Model file for the job. Use its own axes, mm. A direction names the side the tool comes from. Give positions to 0.01 mm unless a question says otherwise; leave off trailing zeros. Loops run counter-clockwise (first coordinate to the right, second up) from the corner with the lowest first, then second, coordinate; pieces in that order, holes last. Notation, with made-up numbers: M -14.5,-37 L 39.5,-37 A23 cw 39.5,-3 Z; hole C 27.25,58.5 d4. An arc over 180 degrees is marked long. Answer in a Markdown table with one row per item.
```python
from build123d import *

# Parameters (mm, degrees)
REVOLUTION001_ANGLE = 16
FILLET_R            = 6


with BuildPart() as part:
    # Sketch → Revolution (revolve)
    with BuildSketch(Plane.XZ):
        with BuildLine():
            ThreePointArc((42.295694, 49.859657), (40.314757, 47.066424), (39.35, 43.780773))
            Line((44.35, 43.780773), (39.35, 43.780773))
            Line((47.827156, 53.147992), (44.35, 43.780773))
            Line((42.827156, 53.147992), (47.827156, 53.147992))
            Line((42.827156, 51.147992), (42.827156, 53.147992))
            ThreePointArc((42.295694, 49.859657), (42.689073, 50.451167), (42.827156, 51.147992))
        make_face()
    revolve(axis=Axis((0, 0, 0), (0, 0, 1)))

    # Sketch004 → Revolution001 (revolve, symmetric)
    with BuildSketch(Plane.XZ) as revolution001_sk:
        with BuildLine():
            Line((44.35, 43.780773), (44.072018, 50.32))
            Line((44.072018, 50.32), (47.83229, 53.160461))
            Line((47.83229, 53.160461), (50.83229, 53.160461))
            Line((50.83229, 53.160461), (50.83229, 65.160461))
            Line((50.83229, 65.160461), (60.83229, 65.160461))
            Line((60.83229, 65.160461), (60.83229, 53.160461))
            add(Edge.make_bspline(
                [(50.83229, 43.780773), (60.83229, 43.780773), (60.83229, 53.160461)],
                knots=[4.712389, 4.712389, 4.712389, 6.283185, 6.283185, 6.283185], degree=2, weights=[1, 0.707107, 1]))
            Line((50.83229, 43.780773), (44.35, 43.780773))
        make_face()
    revolve(axis=Axis((0, 0, 0), (0, 0, 1)), revolution_arc=REVOLUTION001_ANGLE / 2)
    revolve(revolution001_sk.sketch, axis=Axis((0, 0, 0), (0, 0, -1)), revolution_arc=REVOLUTION001_ANGLE / 2)

    # Sketch003 → Groove (revolve, cut)
    with BuildSketch(Plane(origin=(51, 0, 59), x_dir=(-1, 0, 0), z_dir=(0, -1, 0))):
        Polygon((0, 5), (-2, 2.25), (-42.222773, 2.25), (-42.222773, 0), (36.192486, 0), (36.192486, 5), align=None)
    revolve(axis=Axis((51, 0, 59), (-1, 0, 0)), mode=Mode.SUBTRACT)

    # Fillet
    fillet_edges = [part.edges().sort_by_distance(p)[0] for p in [
        (55.288934, -7.770353, 65.160461),
        (55.288934, 7.770353, 65.160461),
    ]]
    fillet(fillet_edges, radius=FILLET_R)


solid = part.part
```
(1) Saw through at A-A, the plane x = 0. Give the cut face in (y, z).
Established:
| item | result |
|---|---|
| outline | M -47.83,53.15 L -44.35,43.78 L -39.35,43.78 A10.38 ccw -42.3,49.86 A1.83 cw -42.83,51.15 L -42.83,53.15 Z; M 39.35,43.78 L 44.35,43.78 L 47.83,53.15 L 42.83,53.15 L 42.83,51.15 A1.83 cw 42.3,49.86 A10.38 ccw Z |
(2) Mould opens along Z. For faces 6 (the flat face through (54.01, 7.59, 51.58)), 7 (the cylindrical face through (56.971, -0.099, 61.248)), 8 (the cylindrical face through (55.44, -5.97, 63.45)) say: pulls with the +Z half, pulls with the -Z half, needs draft (parallel to the pull), parting line crosses it, or undercut.
Established:
| item | result |
|---|---|
| face 6 | needs draft |
| face 7 | undercut |
| face 8 | pulls with the +Z half |
(3) Which spindle directions (+Z, -Z, +X, -X, +Y, -Y) get a long thin tool onto all of the face, cutting with end or side? Do faces 1 (the cylindrical face through (-5.575, 42.463, 52.162)), 2 (the flat face through (17, 36, 43.781)), 3 (the conical face through (52.903, -0.716, 56.727)), 4 (the flat face through (17.9, 39.2, 53.148)), 5 (the cylindrical face through (50.805, 1.676, 53.911)). Say none if no direction does.
Established:
| item | result |
|---|---|
| face 1 | +Z |
| face 2 | -Z, +X, -X, +Y, -Y |
| face 3 | -X |
| face 4 | +Z, -X, +Y, -Y |
| face 5 | +Z, -X |
(4) Flat gauge pins, fed straight in: P1, Ø7, axis at y = 0, z = 59, coming from the -X side; P2, Ø3, axis at y = 16, z = 50, coming from the -X side; P3, Ø2, axis at x = -25.5, z = 50.5, coming from the -Y side. Where does each tip first touch, or does it go through?
Established:
| item | result |
|---|---|
| P1 | stops at x = 52.09 |
| P2 | stops at x = -44.62 |
| P3 | stops at y = -40.07 |
(5) Wall check: L1, parallel to Z at x = 50.7, y = 0; L2, parallel to Y at x = 57, z = 59; L3, parallel to Y at x = 58.5, z = 59. Give the ranges that are in metal, low to high.
Established:
| item | result |
|---|---|
| L1 | z = 43.78 to 53.16 |
| L2 | y = -8.01 to -2.25, 2.25 to 8.01 |
| L3 | y = -8.22 to -2.25, 2.25 to 8.22 |
